```python
from build123d import *

# Parameters (mm, degrees)
SKETCH_1_W          = 38
SKETCH_1_H          = 50
EXTRUDE_1_DEPTH     = 10
CHAMFER_1_SIZE      = 5
CUT_EXTRUDE_1_REACH = 34.955
SKETCH_2_R          = 2.1


with BuildPart() as part:
    # 草圖1 → 填料-伸長1 (new body)
    with BuildSketch(Plane.XY):
        Rectangle(SKETCH_1_W, SKETCH_1_H)
    extrude(amount=EXTRUDE_1_DEPTH)

    # 導角1
    chamfer_1_edges = [part.edges().sort_by_distance(p)[0] for p in [
        (19, -25, 5),
        (-19, -25, 5),
        (-19, 25, 5),
        (19, 25, 5),
    ]]
    chamfer(chamfer_1_edges, length=CHAMFER_1_SIZE)

    # 草圖2 → 除料-伸長1 (cut, up to next)
    with BuildSketch(Plane(origin=(0, 0, 0), x_dir=(-1, 0, 0), z_dir=(0, 0, -1)), mode=Mode.PRIVATE) as cut_extrude_1_sk1:
        with Locations((-10, 17.5)):
            Circle(SKETCH_2_R)
    cut_extrude_1_tool1 = extrude(cut_extrude_1_sk1.sketch, amount=-CUT_EXTRUDE_1_REACH, mode=Mode.PRIVATE) & part.part
    # 草圖2 → 除料-伸長1 (cut, up to next)
    with BuildSketch(Plane(origin=(0, 0, 0), x_dir=(-1, 0, 0), z_dir=(0, 0, -1)), mode=Mode.PRIVATE) as cut_extrude_1_sk2:
        with Locations((10, 17.5)):
            Circle(SKETCH_2_R)
    cut_extrude_1_tool2 = extrude(cut_extrude_1_sk2.sketch, amount=-CUT_EXTRUDE_1_REACH, mode=Mode.PRIVATE) & part.part
    # 草圖2 → 除料-伸長1 (cut, up to next)
    with BuildSketch(Plane(origin=(0, 0, 0), x_dir=(-1, 0, 0), z_dir=(0, 0, -1)), mode=Mode.PRIVATE) as cut_extrude_1_sk3:
        with Locations((-10, -17.5)):
            Circle(SKETCH_2_R)
    cut_extrude_1_tool3 = extrude(cut_extrude_1_sk3.sketch, amount=-CUT_EXTRUDE_1_REACH, mode=Mode.PRIVATE) & part.part
    # 草圖2 → 除料-伸長1 (cut, up to next)
    with BuildSketch(Plane(origin=(0, 0, 0), x_dir=(-1, 0, 0), z_dir=(0, 0, -1)), mode=Mode.PRIVATE) as cut_extrude_1_sk4:
        with Locations((10, -17.5)):
            Circle(SKETCH_2_R)
    cut_extrude_1_tool4 = extrude(cut_extrude_1_sk4.sketch, amount=-CUT_EXTRUDE_1_REACH, mode=Mode.PRIVATE) & part.part
    add(cut_extrude_1_tool1.solids().sort_by_distance((10, 17.5, 0))[0], mode=Mode.SUBTRACT)
    add(cut_extrude_1_tool2.solids().sort_by_distance((-10, 17.5, 0))[0], mode=Mode.SUBTRACT)
    add(cut_extrude_1_tool3.solids().sort_by_distance((10, -17.5, 0))[0], mode=Mode.SUBTRACT)
    add(cut_extrude_1_tool4.solids().sort_by_distance((-10, -17.5, 0))[0], mode=Mode.SUBTRACT)


solid = part.part
```
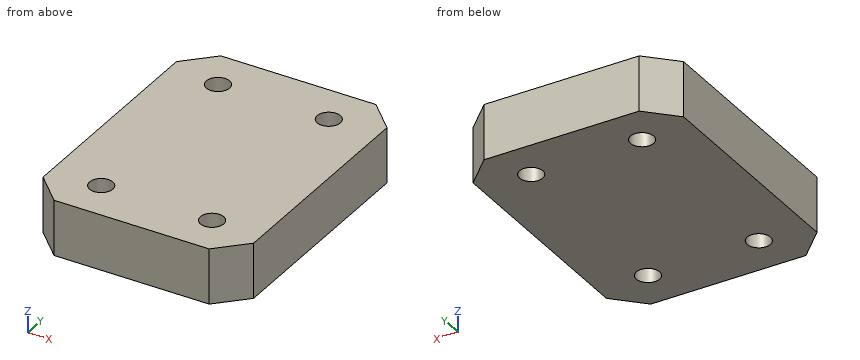
For this review, take the finished solid that the model builds, in its own axes (mm). Give positions to 0.01 mm unless a question says otherwise; leave off trailing zeros. Loops run counter-clockwise (first coordinate to the right, second up) from the corner with the lowest first, then second, coordinate; pieces in that order, holes last. Notation, with made-up numbers: M -37,60 L -15,60 A9 ccw -15,67 Z; hole C 18,15 d10. An arc over 180 degrees is marked long. One line per item, written item: value. Start each with the question number.
Q1. Add section C-C (z = 5.75). Give the boundary of the cut face in (x, y).
Q2. Add section B-B (x = -10). Give the boundary of the cut face in (y, z).
Q3. For L1, parallel to Y at x = 10, z = 8.25; L2, parallel to Y at x = -9, z = 8.5; L3, parallel to Y at x = -15.5, z = 5, list the stretches that pass through material, from the lowest coordinate up.
Q4. Add section A-A (y = 17.5). Give the boundary of the cut face in (x, z).
Reply:
1. outline: M -19,-20 L -14,-25 L 14,-25 L 19,-20 L 19,20 L 14,25 L -14,25 L -19,20 Z; hole C -10,-17.5 d4.2; hole C -10,17.5 d4.2; hole C 10,-17.5 d4.2; hole C 10,17.5 d4.2
2. outline: M -25,0 L -19.6,0 L -19.6,10 L -25,10 Z; M -15.4,0 L 15.4,0 L 15.4,10 L -15.4,10 Z; M 19.6,0 L 25,0 L 25,10 L 19.6,10 Z
3. L1: -25 to -19.6, -15.4 to 15.4, 19.6 to 25
3. L2: -25 to -19.35, -15.65 to 15.65, 19.35 to 25
3. L3: -23.5 to 23.5
4. outline: M -19,0 L -12.1,0 L -12.1,10 L -19,10 Z; M -7.9,0 L 7.9,0 L 7.9,10 L -7.9,10 Z; M 12.1,0 L 19,0 L 19,10 L 12.1,10 Z
